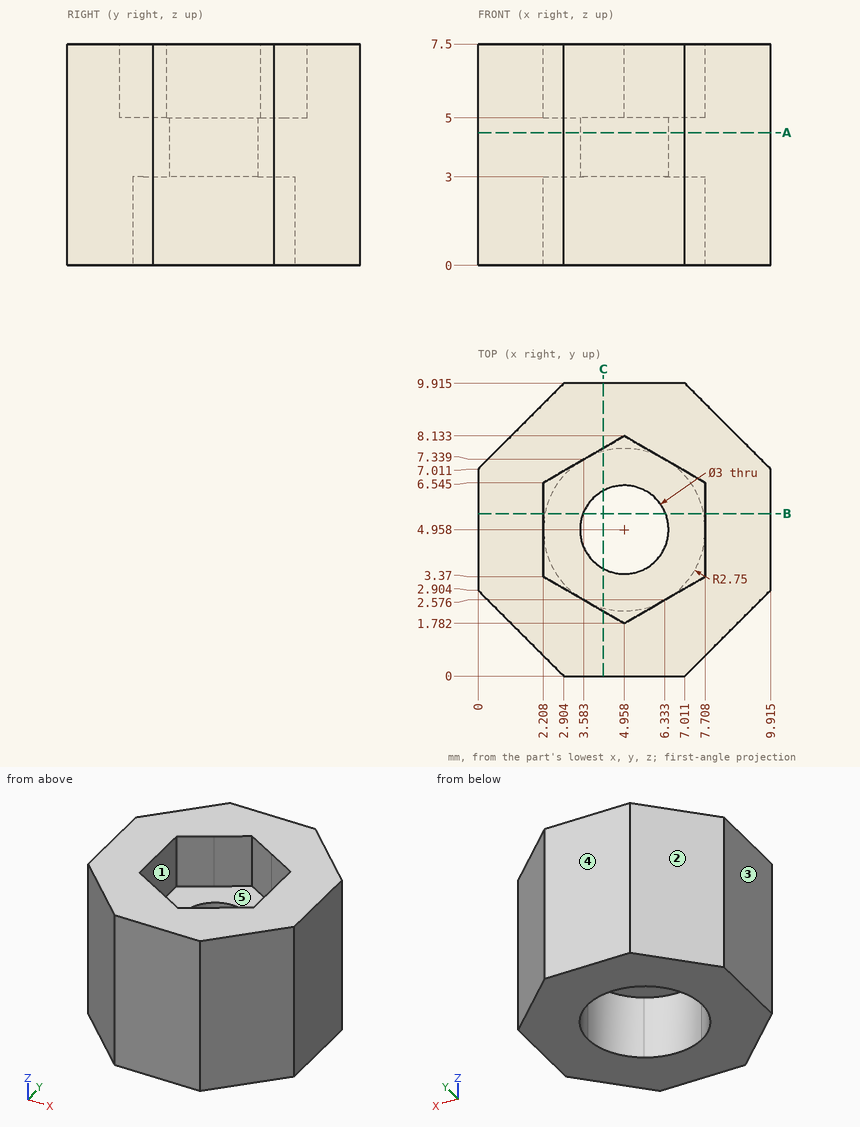
Part print with two shaded views. Sizes in mm from the minimum x, y, z corner. A direction names the side the tool comes from. Give positions to 0.01 mm unless a question says otherwise; leave off trailing zeros. Loops run counter-clockwise (first coordinate to the right, second up) from the corner with the lowest first, then second, coordinate; pieces in that order, holes last. Notation, with made-up numbers: (37.5, -26.5) - (49.5, -26.5) arc R6 ccw to (49.5, -22.5) - close; hole circle Ø3 at (25.25, 82.25). An arc over 180 degrees is marked (long way). Put each result on its own line as item: value.
Q1. Mould opens along Y. For the marked faces 1, 2 and 3 say: pulls with the +Y half, pulls with the -Y half, needs draft (parallel to the pull), parting line crosses it, or undercut.
Filled in:
face 1: undercut
face 2: pulls with the +Y half
face 3: needs draft
Q2. Slice it at A-A (z = 4.5). Give the cut face in (x, y) (1 decimal).
Filled in:
outline: (0, 2.9) - (2.9, 0) - (7, 0) - (9.9, 2.9) - (9.9, 7) - (7, 9.9) - (2.9, 9.9) - (0, 7) - close; hole circle Ø3 at (5, 5)
Q3. Slice it at C-C (x = 4.25). Give the cut face in (y, z) (1 decimal).
Filled in:
outline: (0, 0) - (2.3, 0) - (2.3, 3) - (3.6, 3) - (3.6, 5) - (2.2, 5) - (2.2, 7.5) - (0, 7.5) - close; (6.3, 3) - (7.6, 3) - (7.6, 0) - (9.9, 0) - (9.9, 7.5) - (7.7, 7.5) - (7.7, 5) - (6.3, 5) - close
Q4. Flat gauge pins, fed straight in: pin 1 (3 mm diameter, centred on x = 4, y = 5.5, fed in from +Z); pin 2 (1 mm diameter, centred on y = 8, z = 2, fed in from -X). Where does each tip first touch, or does it go through?
Filled in:
pin 1: stops at z = 5
pin 2: stops at x = 0.49
Q5. Tool access for the marked faces 4 and 5: list every direction of +Z, -Z, +X, -X, +Y, -Y with a clear straight run to the whole face (end or side of a thin tool).
Filled in:
face 4: +Z, -Z, +X, -X, +Y
face 5: +Z
Q6. Slice it at B-B (y = 5.5). Give the cut face in (x, z) (1 decimal).
Filled in:
outline: (0, 0) - (2.3, 0) - (2.3, 3) - (3.6, 3) - (3.6, 5) - (2.2, 5) - (2.2, 7.5) - (0, 7.5) - close; (6.4, 3) - (7.7, 3) - (7.7, 0) - (9.9, 0) - (9.9, 7.5) - (7.7, 7.5) - (7.7, 5) - (6.4, 5) - close
Q7. Probe line 1 along X through (y, z) = (6, 7.25) (1 decimal); line 2 along Z through (x, y) = (3.75, 3.75); line 3 along Y through (x, z) = (2.75, 2.5) (1 decimal). List the from-to ranges inside material, lowest first.
Filled in:
line 1: x = 0 to 2.2, 7.7 to 9.9
line 2: z = 3 to 5
line 3: y = 0.2 to 3.3, 6.6 to 9.8
